from build123d import *

# Parameters (mm, degrees)
F0_W         = 50
F0_H         = 15
F1_DEPTH     = 30
F2_R         = 5
F3_T1_DEPTH  = 52.5
F3_T3_DEPTH  = 5
F3_T5_DEPTH  = 32.5
F3_S9_W      = 5.1
F3_S9_H      = 5.1
F3_T10_DEPTH = 5.1
F3_S15_W     = 5.1
F3_S15_H     = 5.1
F3_T16_DEPTH = 5.1
F4_DEPTH     = 20
F1_FACE1_W   = 20
F1_FACE1_H   = 5
F5_DEPTH     = 57.6854757965
F5_TAPER     = -15


# Not quite as in the source:
# - a fillet or chamfer that OpenCascade refuses, or shapes differently, is made with other operations: its cross-section is extruded or revolved along the edge and cut away or added


with BuildPart() as f1:
    # F0 (on Front) → F1 (new body)
    with BuildSketch(Plane.XZ):
        with Locations((-8.187652571, -9.1238242388)):
            Rectangle(F0_W, F0_H)
    extrude(amount=F1_DEPTH)

    # F2
    f2_edges = [f1.edges().sort_by_distance(p)[0] for p in [
        (16.812347, -15, -16.623824),
        (16.812347, -15, -1.623824),
        (16.812347, 0, -9.123824),
        (16.812347, -30, -9.123824),
        (-8.187653, -30, -16.623824),
        (-8.187653, -30, -1.623824),
        (-33.187653, -30, -9.123824),
    ]]
    fillet(f2_edges, radius=F2_R)

    # F3: fillet of radius 5 on 7 edges, made by hand

    # F3_s2 → F3_t1 (cut)
    with BuildSketch(Plane.YZ.offset(-28.187652571)):
        with BuildLine():
            ThreePointArc((-5, -16.6238242388), (-1.4644660941, -15.1593581447), (0, -11.6238242388))
            Line((0, -11.6238242388), (0, -16.6238242388))
            Line((0, -16.6238242388), (-5, -16.6238242388))
        make_face()
        with BuildLine():
            ThreePointArc((0, -6.6238242388), (-1.4644660941, -3.0882903328), (-5, -1.6238242388))
            Line((-5, -1.6238242388), (0, -1.6238242388))
            Line((0, -1.6238242388), (0, -6.6238242388))
        make_face()
    extrude(amount=F3_T1_DEPTH, mode=Mode.SUBTRACT)

    # F3_s4 → F3_t3 (cut)
    with BuildSketch(Plane.XY.offset(-11.6238242388)):
        with BuildLine():
            ThreePointArc((-33.187652571, -5), (-31.7231864769, -1.4644660941), (-28.187652571, 0))
            Line((-28.187652571, 0), (-33.187652571, 0))
            Line((-33.187652571, 0), (-33.187652571, -5))
        make_face()
    extrude(amount=F3_T3_DEPTH, mode=Mode.SUBTRACT)

    # F3_s6 → F3_t5 (cut)
    with BuildSketch(Plane.XZ.offset(5)):
        with BuildLine():
            ThreePointArc((-33.187652571, -6.6238242388), (-31.7231864769, -3.0882903328), (-28.187652571, -1.6238242388))
            Line((-28.187652571, -1.6238242388), (-33.187652571, -1.6238242388))
            Line((-33.187652571, -1.6238242388), (-33.187652571, -6.6238242388))
        make_face()
        with BuildLine():
            ThreePointArc((-28.187652571, -16.6238242388), (-31.7231864769, -15.1593581447), (-33.187652571, -11.6238242388))
            Line((-33.187652571, -11.6238242388), (-33.187652571, -16.6238242388))
            Line((-33.187652571, -16.6238242388), (-28.187652571, -16.6238242388))
        make_face()
    extrude(amount=F3_T5_DEPTH, mode=Mode.SUBTRACT)


with BuildPart() as f3_tool8:
    # F3_s9 → F3_t10 (new body)
    with BuildSketch(Plane.XY.offset(-11.6238242388)):
        with Locations((-30.737652571, -2.45)):
            Rectangle(F3_S9_W, F3_S9_H)
    extrude(amount=-F3_T10_DEPTH)

    # F3_s11 → F3_t12 (revolve, cut)
    with BuildSketch(Plane(origin=(-28.187652571, -5, -11.6238242388), x_dir=(0.7071067812, -0.7071067812, 0), z_dir=(0.7071067812, 0.7071067812, 0))):
        with BuildLine():
            ThreePointArc((0, -5), (5, 0), (0, 5))
            Line((0, 5), (0, -5))
        make_face()
    revolve(axis=Axis((-28.187652571, -5, -11.6238242388), (0, 0, -1)), mode=Mode.SUBTRACT)


with BuildPart() as f1_1:
    add(f1.part)

    # F3_t7: cut F3_tool8
    add(f3_tool8.part, mode=Mode.SUBTRACT)


with BuildPart() as f3_tool14:
    # F3_s15 → F3_t16 (new body)
    with BuildSketch(Plane.YZ.offset(-28.187652571)):
        with Locations((-2.45, -4.0738242388)):
            Rectangle(F3_S15_W, F3_S15_H)
    extrude(amount=-F3_T16_DEPTH)

    # F3_s17 → F3_t18 (revolve, cut)
    with BuildSketch(Plane(origin=(-28.187652571, -5, -6.6238242388), x_dir=(0, -0.7071067812, -0.7071067812), z_dir=(0, 0.7071067812, -0.7071067812))):
        with BuildLine():
            ThreePointArc((0, -5), (5, 0), (0, 5))
            Line((0, 5), (0, -5))
        make_face()
    revolve(axis=Axis((-28.187652571, -5, -6.6238242388), (-1, 0, 0)), mode=Mode.SUBTRACT)


with BuildPart() as f1_2:
    add(f1_1.part)

    # F3_t13: cut F3_tool14
    add(f3_tool14.part, mode=Mode.SUBTRACT)

    # F4 (cut): a face of the model
    f4_faces = [f1_2.faces().sort_by_distance(p)[0] for p in [
        (16.812347429, -15, -9.1238242388),
    ]]
    extrude(f4_faces, amount=-F4_DEPTH, mode=Mode.SUBTRACT)

    # F1_face1 (on face) → F5 (cut)
    with BuildSketch(Plane(origin=(-33.187652571, -15, -9.1238242388), x_dir=(0, -1, 0), z_dir=(-1, 0, 0))):
        Rectangle(F1_FACE1_W, F1_FACE1_H)
    extrude(amount=-F5_DEPTH, taper=F5_TAPER, mode=Mode.SUBTRACT)


solid = f1_2.part
Check sheet for the modelled part. Datum: model origin and axes. Units: mm. Round coordinates to 2 decimals unless told otherwise and drop trailing zeros. Return JSON: item names as keys, results as strings.
Q1. Depth check by flat-ended pin: P1, Ø2, axis at y = -10, z = -7.5, coming from the -X side; P2, Ø1, axis at x = -23, z = -13, coming from the +Y side; P3, Ø2, axis at y = -7, z = -14.5, coming from the -X side. Enter the tip coordinate at first touch or a pass-through.
Returned:
{"P1": "stops at x = -33.19", "P2": "stops at y = -0.08", "P3": "stops at x = -32.82"}
Q2. Scan lines: L1, parallel to Z at x = -23.5, y = -16.5; L2, parallel to Z at x = -20, y = -8.5; L3, parallel to Y at x = -25, z = -11. Record each from-to range of solid material in increasing order. Write a range as from..to.
Returned:
{"L1": "z = -16.62..-14.22, -4.03..-1.62", "L2": "z = -16.62..-15.16, -3.09..-1.62", "L3": "y = -30..-27.19, -2.81..0"}
Q3. Cross-section at A-A (x = -17.5). Give the number of separate pieces and of enclosed holes in the cut face, then the cut area to 3 significant figures.
Returned:
{"separate pieces": "4", "enclosed holes": "0", "area": "51.5 mm²"}
